Geometry: final body of the model. Coordinates: model frame, mm. A direction names the side the tool comes from. Coordinates: 2 decimals unless noted, no trailing zeros. Loops run counter-clockwise (first coordinate to the right, second up) from the corner with the lowest first, then second, coordinate; pieces in that order, holes last. Notation, with made-up numbers: (-20.5, 21) - (22.5, 21) arc R18 cw to (22.5, 35) - close; hole circle Ø2 at (-7.75, 36.5). An arc over 180 degrees is marked (long way). Write each question's results on one line, items separated by ' | '. Start each with the question number.
from build123d import *


with BuildPart() as f1:
    # F0 (on Front) → F1 (revolve)
    with BuildSketch(Plane.XZ):
        with BuildLine():
            Line((27.5, 23.5), (27.5, 27.5))
            Line((27.5, 27.5), (2.864325, 29.862948))
            ThreePointArc((2.864325, 29.862948), (1.433801, 29.965717), (0, 30))
            ThreePointArc((0, 30), (-1.433801, 29.965717), (-2.864325, 29.862948))
            Line((-2.864325, 29.862948), (-27.5, 27.5))
            Line((-27.5, 27.5), (-27.5, 23.5))
            Line((-27.5, 23.5), (-13.5, 23.5))
            Line((-13.5, 23.5), (-13.5, 12))
            Line((-13.5, 12), (0, 12))
            Line((0, 12), (13.5, 12))
            Line((13.5, 12), (13.5, 23.5))
            Line((13.5, 23.5), (27.5, 23.5))
        make_face()
    revolve(axis=Axis((13.75, 0, 0), (1, 0, 0)))


solid = f1.part
1) Pin query (flat end, axial travel): pin 1 Ø10 at (y, z) = (2.5, 22.5) entering from -X; pin 2 Ø12 at (y, z) = (-12.5, -6) entering from +X; pin 3 Ø1.5 at (x, y) = (-19, 10) entering from +Z; pin 4 Ø4 at (x, z) = (6.5, -10) entering from +Y. Return the tip coordinate at first contact, or that it passes through.
2) Pull-direction query (Y, two-part tool) for faces 1 (the flat face through (-27.5, -12.4, 20.2)), 2 (the cylindrical face through (20.6, -7.1, 22.4)), 3 (the conical face through (-18.092, 27.727, -6.157)); classes: released by +Y, released by -Y, zero draft, split by the parting line, or undercut.
3) Material intervals for line 1 (Y direction, x = 19.5, z = 0); line 2 (Y direction, x = -17.5, z = 0); line 3 (Z direction, x = 18.5, y = -13), sorted ascending. Write a range as [from, to].
4) Section query A-A on x = 18.5. Output: boundary loops of the cut face in (y, z).
5) Section query B-B on x = 11. Output: boundary loops of the cut face in (y, z), and give its area (3 significant figures).
6) Access query for faces 4 (the cylindrical face through (0.19, -0.53, -11.99)), 5 (the flat face through (13.5, -6, 11)), 6 (the flat face through (-13.5, -6, -11)). Directions: +Z, -Z, +X, -X, +Y, -Y. A direction counts if a zero-diameter tool reaches every point of the face in a straight line with its end or side. Return the directions, or none.
Returned:
1) pin 1: stops at x = -27.5 | pin 2: stops at x = 13.5 | pin 3: stops at z = 26.77 | pin 4: stops at y = 28.44
2) face 1: zero draft | face 2: undercut | face 3: split by the parting line
3) line 1: y = [-28.27, -23.5], [23.5, 28.27] | line 2: y = [-28.46, -23.5], [23.5, 28.46] | line 3: z = [-25.21, -19.58], [19.58, 25.21]
4) outline: circle Ø56.73 at (0, 0); hole circle Ø47 at (0, 0)
5) outline: circle Ø58.17 at (0, 0); hole circle Ø24 at (0, 0) | area: 2,200 mm²
6) face 4: +X, -X | face 5: +X | face 6: -X
